Can you work these out from the model? Positions are in its coordinate system, mm. Face numbers are marked on the shaded views. Coordinates: 2 decimals unless noted, no trailing zeros. Order: outer loops, then holes, each group sorted by start corner. A loop starts at its lowest first (then second) coordinate and runs counter-clockwise, first axis right, second up. Notation, with made-up numbers: (55.25, 14.25) -> (113.25, 14.25) arc R13 ccw to (113.25, 29.25) -> close; hole circle Ø2 at (51.25, -32.5). An arc over 180 degrees is marked (long way). Use a Markdown table: item, result. Add a question column.
1. For pin 1 Ø1 at (x, y) = (7, 1) entering from -Z; pin 2 Ø1.5 at (y, z) = (-1, -32) entering from +X; pin 3 Ø1 at (x, y) = (47, 3.5) entering from -Z, each with a flat end and sliding along its axis, tell me the tip position at first contact or that it passes through.
2. If I drill on line 1 along Z through (x, y) = (-39, 0.75); line 2 along Z through (x, y) = (0, -0.5); line 3 along Z through (x, y) = (-39.5, -2.5), over which ranges is the centre line in solid material (lowest first)? Write a range as from..to.
3. We'd pull the mould along X, two halves only. Please class the marked faces 1, 2 and 3: pulls with the +X half, pulls with the -X half, needs draft (parallel to the pull), parting line crosses it, or undercut.
4. Suppose I cut it at B-B, the plane x = 35. List the corners of the cut face in (y, z) for me, then the cut area to 3 significant figures.
5. Suppose I cut it at C-C, the plane z = 33. List the corners of the cut face in (x, y) for me.
6. Suppose I cut it at D-D, the plane y = 0.5. State how many separate pieces and enclosed holes the cut face has, then the cut area to 3 significant figures.
7. Suppose I cut it at A-A, the plane z = 0. List the corners of the cut face in (x, y) for me.
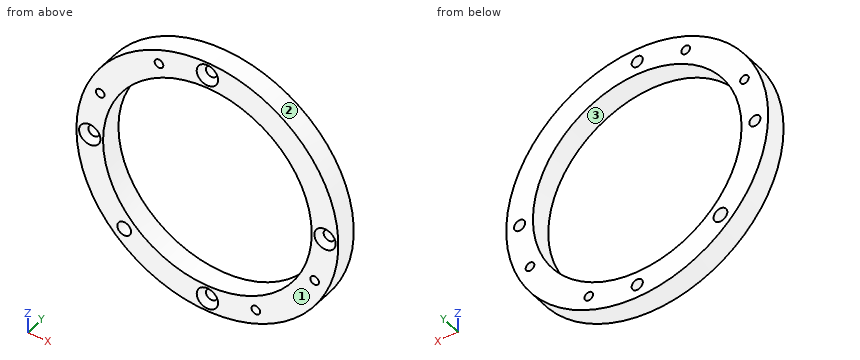
Autodesk Inventor part; units mm, degrees
ref_plane "YZ Plane" through (0, 0, 0) normal (1, 0, 0) x (0, 1, 0)
ref_plane "XZ Plane" through (0, 0, 0) normal (0, 1, 0) x (-1, 0, 0)
ref_plane "XY Plane" through (0, 0, 0) normal (0, 0, 1) x (1, 0, 0)
sketch "Sketch1" plane through (0, 0, 0) normal (0, 1, 0) x (-1, 0, 0)
  circle A0 centre (0, 0) radius 35 construction
  circle A1 centre (0, 0) radius 47.8
  circle A2 centre (0, 0) radius 60
  line L0 (0, -35) -> (0, -60) construction
  point P0 (0, -47.5)
  dimension "d0" = 70
  dimension "d1" = 120
  dimension "d42" = 12.2
extrude "Extrusion1" add sketch "Sketch1" along normal mid plane 10
sketch "Sketch3" plane through (0, -5, 0) normal (0, -1, 0) x (1, 0, 0)
  circle A0 centre (0, 0) radius 47.8 construction
  circle A1 centre (0, 0) radius 60 construction
  circle A2 centre (0, 0) radius 47.8 construction
  line L0 (47.8, 0) -> (60, 0) construction
  circle A3 centre (0, 0) radius 47.8 construction
  circle A4 centre (0, 0) radius 60 construction
  point P0 (53.9, 0)
  dimension "d43" = 120
  dimension "d44" = 53.9
hole "Hole2" at (53.9, -5, 0) direction (0, 1, 0) diameter 5.1054 end through all countersink diameter 9.779 countersink angle 82
pattern_circular "Circular Pattern2" count 4 over 360 about axis through (0, 0, 0) along (0, 1, 0) of "Hole2"
sketch "Sketch4" plane through (0, 5, 0) normal (0, 1, 0) x (1, 0, 0)
  line L0 (22.1829, 49.1236) -> (-49.1236, -22.1829) construction
  line L1 (-49.1236, -22.1829) -> (-22.1829, -49.1236) construction
  line L2 (-22.1829, -49.1236) -> (49.1236, 22.1829) construction
  line L3 (49.1236, 22.1829) -> (22.1829, 49.1236) construction
  line L4 (22.1829, 49.1236) -> (-22.1829, -49.1236) construction
  line L5 (-49.1236, -22.1829) -> (49.1236, 22.1829) construction
  circle A0 centre (0, -53.9) radius 2.5527 construction
  circle A1 centre (-53.9, 0) radius 2.5527 construction
  circle A2 centre (0, 53.9) radius 2.5527 construction
  circle A3 centre (53.9, 0) radius 2.5527 construction
  circle A4 centre (0, 0) radius 47.8 construction
  circle A5 centre (0, 0) radius 60 construction
  circle A6 centre (0, 53.9) radius 2.5527 construction
  circle A7 centre (0, 0) radius 53.9 construction
  circle A8 centre (53.9, 0) radius 2.5527 construction
  line L6 (0, 0) -> (53.9, 0) construction
  point P0 (49.1236, 22.1829)
  point P1 (-49.1236, -22.1829)
  dimension "d25" = 38.1
  dimension "d26" = 45
hole "Hole3" at (22.1829, 5, -49.1236) at (49.1236, 5, -22.1829) at (-49.1236, 5, 22.1829) at (-22.1829, 5, 49.1236) direction (0, -1, 0) diameter 3.9624 end through all
sketch "Sketch5" plane through (0, 5, 0) normal (0, 1, 0) x (1, 0, 0)
  circle A0 centre (0, 0) radius 60 construction
  line L0 (-42.4264, 42.4264) -> (-33.7997, 33.7997) construction
  circle A1 centre (0, 0) radius 47.8 construction
  circle A2 centre (-53.9, 0) radius 2.5527 construction
  circle A3 centre (53.9, 0) radius 2.5527 construction
  line L1 (-53.9, 0) -> (53.9, 0) construction
  point P0 (-38.1131, 38.1131)
  point P1 (-38.1131, 38.1131)
  dimension "d34" = 45
hole "Hole4" at (-38.1131, 5, -38.1131) direction (0, -1, 0) diameter 6.3246 end through all
properties part number "4in LS-002" material "Aluminum 6061"
Worked out:
| question | item | result |
|---|---|---|
| 1 | pin 1 | stops at z = -59.65 |
| 1 | pin 2 | stops at x = 51.22 |
| 1 | pin 3 | stops at z = -37.92 |
| 2 | line 1 | z = -45.6..-41.15, -35.08..-27.64, 27.64..45.6 |
| 2 | line 2 | z = -60..-56.45, -51.35..-47.8, 47.8..51.35, 56.45..60 |
| 2 | line 3 | z = -45.16..-40.96, -35.27..-26.92, 26.92..45.16 |
| 3 | face 1 | needs draft |
| 3 | face 2 | parting line crosses it |
| 3 | face 3 | undercut |
| 4 | outline | (-5, -48.73) -> (5, -48.73) -> (5, -32.56) -> (-5, -32.56) -> close; (-5, 32.56) -> (5, 32.56) -> (5, 48.73) -> (-5, 48.73) -> close |
| 4 | area | 324 mm² |
| 5 | outline | (-50.11, -5) -> (-34.58, -5) -> (-34.58, 5) -> (-50.11, 5) -> close; (34.58, -5) -> (50.11, -5) -> (50.11, 5) -> (34.58, 5) -> close |
| 6 | separate pieces | 1 |
| 6 | enclosed holes | 10 |
| 6 | area | 3,970 mm² |
| 7 | outline | (-60, -5) -> (-58.79, -5) -> (-56.45, -2.31) -> (-56.45, 5) -> (-60, 5) -> close; (-51.35, -2.31) -> (-49.01, -5) -> (-47.8, -5) -> (-47.8, 5) -> (-51.35, 5) -> close; (47.8, -5) -> (49.01, -5) -> (51.35, -2.31) -> (51.35, 5) -> (47.8, 5) -> close; (56.45, -2.31) -> (58.79, -5) -> (60, -5) -> (60, 5) -> (56.45, 5) -> close |
